Autodesk Inventor part; units mm, degrees
ref_plane "YZ Plane" through (0, 0, 0) normal (1, 0, 0) x (0, 1, 0)
ref_plane "XZ Plane" through (0, 0, 0) normal (0, 1, 0) x (-1, 0, 0)
ref_plane "XY Plane" through (0, 0, 0) normal (0, 0, 1) x (1, 0, 0)
sketch "Náčrt1" plane through (0, 0, 0) normal (0, 0, 1) x (1, 0, 0)
  line L0 (0, 0) -> (30, 0)
  line L1 (30, 0) -> (30, 2)
  line L2 (30, 2) -> (16, 2)
  line L3 (16, 2) -> (16, 30)
  line L4 (16, 30) -> (14, 30)
  line L5 (14, 30) -> (14, 2)
  line L6 (14, 2) -> (0, 2)
  line L7 (0, 2) -> (0, 0)
  dimension "d0" = 30
  dimension "d1" = 2
  dimension "d2" = 14
  dimension "d3" = 28
  dimension "d4" = 2
extrude "Vysunutí1" add sketch "Náčrt1" along normal blind 1200
sketch "Náčrt2" plane through (16, 2, 0) normal (0, 1, 0) x (1, 0, 0)
  line L0 (0, 0) -> (0, -1200)
  line L1 (14, -1200) -> (0, -1200)
  circle A0 centre (7, -1185) radius 1.5
  line L2 (14, 0) -> (14, -1200)
  line L3 (14, -600) -> (0, -600)
  circle A1 centre (7, -15) radius 1.5
  point P0 (-16, 0)
  dimension "d7" = 15
  dimension "d8" = 3
extrude "Vysunutí2" cut sketch "Náčrt2" against normal up to next contours A0 | A1
equation "\"d0\" = width_A"
equation "\"d2\" = -0.5 * thickness + 0.5 * width_A"
equation "\"d3\" = width_B - thickness"
equation "\"d4\" = thickness"
equation "\"d5\" = length"
equation "\"d7\" = 0.5 * gSquareProfile_Width_Rack"
equation "\"width_A\" = 30"
equation "\"width_B\" = 30"
equation "\"thickness\" = 2"
equation "\"length\" = gRack_Cpu_Length"
properties part number "Profile-T#01"
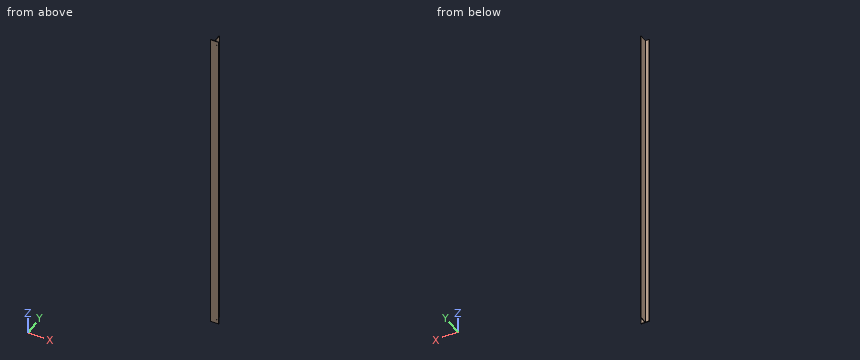
Design review of the part built by this model. Coordinates are the model's own, in mm. Coordinates: 2 decimals unless noted, no trailing zeros. Loops run counter-clockwise (first coordinate to the right, second up) from the corner with the lowest first, then second, coordinate; pieces in that order, holes last.
Item 1: Add section C-C (y = 11.75). Write out the cut boundary in (x, z).
Completed:
outline: (14, 0) - (16, 0) - (16, 1200) - (14, 1200) - close
Item 2: Add section B-B (x = 5.75). Write out the cut boundary in (y, z).
Completed:
outline: (0, 0) - (2, 0) - (2, 1200) - (0, 1200) - close
Item 3: Wall thickness on L1, parallel to Z at x = 23, y = 1.2; L2, parallel to X at y = 0.85, z = 15; L3, parallel to Y at x = 13.5, z = 781.5: over which ranges is each line inside the solid? List them lowest first.
Completed:
L1: z = 0 to 13.5, 16.5 to 1183.5, 1186.5 to 1200
L2: x = 0 to 21.5, 24.5 to 30
L3: y = 0 to 2
Item 4: Clearance check with flat-ended pins moving along their axes: pin 1 (5 mm diameter, centred on x = 23, z = 1185, fed in from -Y); pin 2 (7 mm diameter, centred on x = 20.5, z = 745, fed in from +Y); pin 3 (14 mm diameter, centred on y = 21, z = 777.5, fed in from +X); pin 4 (5 mm diameter, centred on y = 12.5, z = 359.5, fed in from -X). State where each tip first meets the part, or that it passes through.
Completed:
pin 1: stops at y = 0
pin 2: stops at y = 2
pin 3: stops at x = 16
pin 4: stops at x = 14
Item 5: Add section A-A (z = 358). Write out the cut boundary in (x, y).
Completed:
outline: (0, 0) - (30, 0) - (30, 2) - (16, 2) - (16, 30) - (14, 30) - (14, 2) - (0, 2) - close
